Can you work these out from the model? Positions are in its coordinate system, mm. A direction names the side the tool comes from. Coordinates: 2 decimals unless noted, no trailing zeros. Order: outer loops, then holes, each group sorted by start corner. A loop starts at its lowest first (then second) coordinate and runs counter-clockwise, first axis right, second up. Notation, with made-up numbers: (65, 58.5) -> (104, 58.5) arc R14 ccw to (104, 68.5) -> close; hole circle Ø6 at (-28.75, -14.5). An arc over 180 degrees is marked (long way). Return JSON: item names as keys, results as strings. Group by question number.
1) For pin 1 (5.5 mm diameter, centred on x = -12, y = -70.5, fed in from -Z); pin 2 (9 mm diameter, centred on x = -14.5, y = -72, fed in from +Z); pin 3 (10 mm diameter, centred on x = -26, y = -71.5, fed in from -Z); pin 4 (3 mm diameter, centred on x = 8, z = 30.5, fed in from -Y), each with a flat end and sliding along its axis, tell me the tip position at first contact or that it passes through.
2) For faces 1 (the cylindrical face through (-3.8, -61.56, 35.33)), 2 (the flat face through (16, -70, 1.778)), 3 (the flat face through (0, -36, 0)), which set-ups out of +Z, -Z, +X, -X, +Y, -Y let a thin tool reach every point of the face, with its end or its side?
3) If I drill on probe 1 along Y at (x, z) = (0, 4); probe 2 along X at (y, z) = (-62.23, 8.5); probe 3 along Z at (x, y) = (-19, -73), over which ranges is the centre line in solid material (lowest first)? Write a range as from..to.
4) Thinking about a two-plate mould opening in X: for faces 4 (the flat face through (0, -8, 17.272)), 5 (the cylindrical face through (14.52, -72.68, 18.17)), 6 (the flat face through (0, -85, 19.05)), 7 (the flat face through (-36.491, -25, 9)), which applies, +X half, -X half, draft (parallel to the pull), parting line (faces both ways), or undercut?
5) If we section it at A-A, the plane z = 4.5: Please give me the cut outline in (x, y), then the cut area to 3 significant figures.
6) If we section it at C-C, the plane z = 29: Please give me the cut outline in (x, y), then the cut area to 3 significant figures.
7) If we section it at B-B, the plane y = -10.5: Please give me the cut outline in (x, z).
from build123d import *

# Parameters (mm, degrees)
SKETCH2_R           = 15.24
BOSS_EXTRUDE2_DEPTH = 19.05
SKETCH3_R           = 39.496431486
SKETCH3_R_2         = 35.260007957
CUT_EXTRUDE2_DEPTH  = 1.778
SKETCH4_R           = 31.746180351
SKETCH4_R_2         = 28.068999156
CUT_EXTRUDE3_DEPTH  = 1.778
CUT_EXTRUDE4_START  = -1.778
SKETCH5_R           = 39.496431486
SKETCH5_R_2         = 35.260007957
CUT_EXTRUDE4_DEPTH  = 1.778
CUT_EXTRUDE5_START  = -1.778
SKETCH7_R           = 31.746180351
SKETCH7_R_2         = 28.068999156
CUT_EXTRUDE5_DEPTH  = 1.778
BOSS_EXTRUDE3_START = -6.35
SKETCH9_R           = 15.24
BOSS_EXTRUDE3_DEPTH = 6.35
SKETCH10_R          = 17.526
BOSS_EXTRUDE4_DEPTH = 33.02


with BuildPart() as part:
    # Sketch2 → Boss-Extrude2 (new body)
    with BuildSketch(Plane.XY):
        with BuildLine():
            Line((20.429296249, -72.446914532), (20.429296249, -45.399816154))
            ThreePointArc((20.429296249, -45.399816154), (25.133677026, -34.04243628), (36.4910569, -29.338055504))
            Line((36.4910569, -29.338055504), (36.4910569, -20.532405534))
            ThreePointArc((36.4910569, -20.532405534), (20.935477727, -5.485511485), (0, 0))
            ThreePointArc((0, 0), (-20.935477727, -5.485511485), (-36.4910569, -20.532405534))
            Line((-36.4910569, -20.532405534), (-36.4910569, -29.338055504))
            ThreePointArc((-36.4910569, -29.338055504), (-25.133677026, -34.04243628), (-20.429296249, -45.399816154))
            Line((-20.429296249, -45.399816154), (-20.429296249, -72.446914532))
            ThreePointArc((-20.429296249, -72.446914532), (-12.360356233, -83.33771782), (0, -88.9))
            ThreePointArc((0, -88.9), (12.360356233, -83.33771782), (20.429296249, -72.446914532))
        make_face()
        with Locations(Location((0, -62.23, 0), (0, 0, 180))):
            Circle(SKETCH2_R, mode=Mode.SUBTRACT)
    extrude(amount=BOSS_EXTRUDE2_DEPTH)

    # Sketch3 → Cut-Extrude2 (cut)
    with BuildSketch(Plane.XY.offset(19.05)):
        with Locations((0, -44.45)):
            Circle(SKETCH3_R)
        with Locations((0, -44.45)):
            Circle(SKETCH3_R_2, mode=Mode.SUBTRACT)
    extrude(amount=-CUT_EXTRUDE2_DEPTH, mode=Mode.SUBTRACT)

    # Sketch4 → Cut-Extrude3 (cut)
    with BuildSketch(Plane.XY.offset(19.05)):
        with Locations((0, -44.45)):
            Circle(SKETCH4_R)
        with Locations((0, -44.45)):
            Circle(SKETCH4_R_2, mode=Mode.SUBTRACT)
    extrude(amount=-CUT_EXTRUDE3_DEPTH, mode=Mode.SUBTRACT)

    # Sketch5 → Cut-Extrude4 (cut)
    with BuildSketch(Plane(origin=(0, 0, 0), x_dir=(-1, 0, 0), z_dir=(0, 0, -1)).offset(CUT_EXTRUDE4_START)):
        with Locations((0, -44.45)):
            Circle(SKETCH5_R)
        with Locations((0, -44.45)):
            Circle(SKETCH5_R_2, mode=Mode.SUBTRACT)
    extrude(amount=CUT_EXTRUDE4_DEPTH, mode=Mode.SUBTRACT)

    # Sketch7 → Cut-Extrude5 (cut)
    with BuildSketch(Plane(origin=(0, 0, 0), x_dir=(-1, 0, 0), z_dir=(0, 0, -1)).offset(CUT_EXTRUDE5_START)):
        with Locations((0, -44.45)):
            Circle(SKETCH7_R)
        with Locations((0, -44.45)):
            Circle(SKETCH7_R_2, mode=Mode.SUBTRACT)
    extrude(amount=CUT_EXTRUDE5_DEPTH, mode=Mode.SUBTRACT)

    # Sketch9 → Boss-Extrude3 (add)
    with BuildSketch(Plane.XY.offset(19.05).offset(BOSS_EXTRUDE3_START)):
        with Locations(Location((0, -62.23, 0), (0, 0, 206.225395775))):
            Circle(SKETCH9_R)
    extrude(amount=BOSS_EXTRUDE3_DEPTH)

    # Sketch10 → Boss-Extrude4 (add)
    with BuildSketch(Plane.XY.offset(19.05)):
        with Locations((0, -44.45)):
            Circle(SKETCH10_R)
    extrude(amount=BOSS_EXTRUDE4_DEPTH)


solid = part.part
Result sheet:
{
 "1": {"pin 1": "stops at z = 0", "pin 2": "stops at z = 19.05", "pin 3": "passes through", "pin 4": "stops at y = -60.73"},
 "2": {"face 1": "+Z", "face 2": "-Z", "face 3": "-Z, +X, -X, +Y, -Y"},
 "3": {"probe 1": "y = -88.9..-77.47, -46.99..0", "probe 2": "x = -20.43..-15.24, 15.24..20.43", "probe 3": "z = 0..19.05"},
 "4": {"face 4": "undercut", "face 5": "undercut", "face 6": "draft", "face 7": "-X half"},
 "5": {"outline": "(-36.49, -29.34) arc R16.06 cw to (-20.43, -45.4) -> (-20.43, -72.45) arc R26.85 ccw to (0, -88.9) arc R26.85 ccw to (20.43, -72.45) -> (20.43, -45.4) arc R16.06 cw to (36.49, -29.34) -> (36.49, -20.53) arc R42.69 ccw to (-36.49, -20.53) -> close; hole circle Ø30.48 at (0, -62.23)", "area": "3,300 mm2"},
 "6": {"outline": "circle Ø35.05 at (0, -44.45)", "area": "965 mm2"},
 "7": {"outline": "(-28.04, 0) -> (-20.18, 0) -> (-20.18, 1.78) -> (-9.52, 1.78) -> (-9.52, 0) -> (9.52, 0) -> (9.52, 1.78) -> (20.18, 1.78) -> (20.18, 0) -> (28.04, 0) -> (28.04, 19.05) -> (20.18, 19.05) -> (20.18, 17.27) -> (9.52, 17.27) -> (9.52, 19.05) -> (-9.52, 19.05) -> (-9.52, 17.27) -> (-20.18, 17.27) -> (-20.18, 19.05) -> (-28.04, 19.05) -> close"}
}
